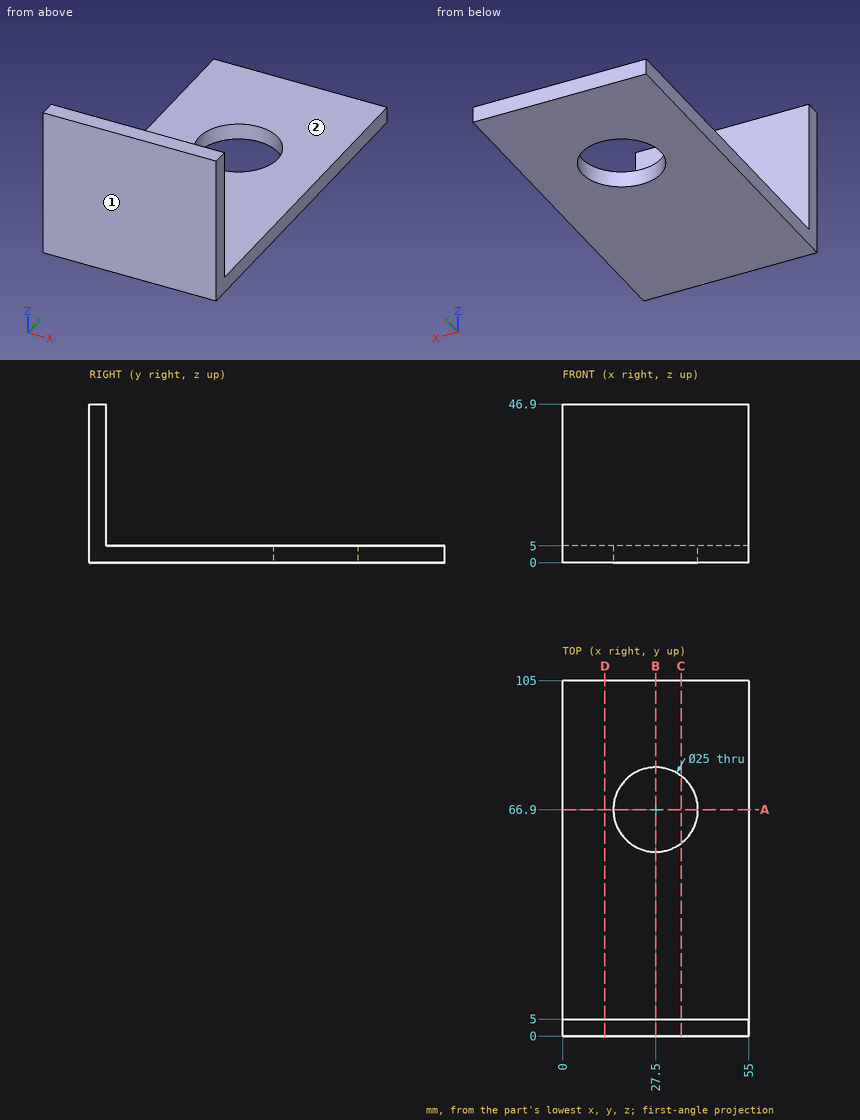
The figure shows three views and two pictorial views of one solid part (mm, origin at its lowest corner). Answer the questions. A direction names the side the tool comes from. Round coordinates to 2 decimals unless told otherwise and drop trailing zeros. Order: outer loops, then holes, each group sorted by start corner. A loop starts at its lowest first (then second) coordinate and runs counter-clockwise, first axis right, second up. Notation, with made-up numbers: (45, 35) -> (64, 35) arc R31 cw to (64, 62) -> close; hole circle Ø2 at (36.25, 44.5). An arc over 180 degrees is marked (long way). One line per item, written item: value.
Item 1: Find section B-B, the plane x = 27.5. Give the vertices of the cut face in (y, z), then the cut area to 4 significant figures.
Taken from the geometry:
outline: (0, 0) -> (54.4, 0) -> (54.4, 5) -> (5, 5) -> (5, 46.9) -> (0, 46.9) -> close; (79.4, 0) -> (105, 0) -> (105, 5) -> (79.4, 5) -> close
area: 609.5 mm2
Item 2: Find section C-C, the plane x = 35. Give the vertices of the cut face in (y, z).
Taken from the geometry:
outline: (0, 0) -> (56.9, 0) -> (56.9, 5) -> (5, 5) -> (5, 46.9) -> (0, 46.9) -> close; (76.9, 0) -> (105, 0) -> (105, 5) -> (76.9, 5) -> close
Item 3: Find section A-A, the plane y = 66.9. Give the vertices of the cut face in (x, z).
Taken from the geometry:
outline: (0, 0) -> (15, 0) -> (15, 5) -> (0, 5) -> close; (40, 0) -> (55, 0) -> (55, 5) -> (40, 5) -> close
Item 4: Find section D-D, the plane x = 12.5. Give the vertices of the cut face in (y, z), then the cut area to 4 significant figures.
Taken from the geometry:
outline: (0, 0) -> (105, 0) -> (105, 5) -> (5, 5) -> (5, 46.9) -> (0, 46.9) -> close
area: 734.5 mm2
Item 5: For the marked faces 1 and 2, determine the directions among +Z, -Z, +X, -X, +Y, -Y from which every point of the face is accessible in a straight line to the end or side of a thin tool.
Taken from the geometry:
face 1: +Z, -Z, +X, -X, -Y
face 2: +Z, +X, -X, +Y
Item 6: Straight lines are drawn through the part: L1, parallel to Y at x = 27.5, z = 3.65; L2, parallel to Y at x = 49.5, z = 40.5. For each, find the intervals that lie inside material, in ascending order.
Taken from the geometry:
L1: y = 0 to 54.4, 79.4 to 105
L2: y = 0 to 5
Item 7: Given P1, Ø16.5, axis at x = 21.5, y = 33.5, coming from the +Z side; P2, Ø10, axis at y = 13.5, z = 42, coming from the +X side; P3, Ø12.5, axis at x = 17, z = 25, coming from the +Y side, each flat-ended and moving along its own axis, determine where each tip first touches the part or whether it passes through.
Taken from the geometry:
P1: stops at z = 5
P2: passes through
P3: stops at y = 5
